Model file for the job. Use its own axes, mm. A direction names the side the tool comes from. Round coordinates to 2 decimals unless told otherwise and drop trailing zeros. Loops run counter-clockwise (first coordinate to the right, second up) from the corner with the lowest first, then second, coordinate; pieces in that order, holes last. Notation, with made-up numbers: (75.5, 27.5) - (119.5, 27.5) arc R17 ccw to (119.5, 39.5) - close; hole circle Ø9 at (81.25, -26). An arc over 180 degrees is marked (long way). Answer as a JSON object with one key per item and string values.
from build123d import *

# Parameters (mm, degrees)
SKETCH1_R           = 2.5
BOSS_EXTRUDE1_DEPTH = 10
SKETCH2_R           = 5
BOSS_EXTRUDE2_DEPTH = 5
FILLET1_R           = 5


with BuildPart() as part:
    # Sketch1 → Boss-Extrude1 (new body)
    with BuildSketch(Plane(origin=(0, 0, 0), x_dir=(1, 0, 0), z_dir=(0, 1, 0))):
        with Locations(Location((0, 0, 0), (0, 0, 270))):
            Circle(SKETCH1_R)
    extrude(amount=-BOSS_EXTRUDE1_DEPTH)

    # Sketch2 → Boss-Extrude2 (add)
    with BuildSketch(Plane(origin=(0, 0, 0), x_dir=(1, 0, 0), z_dir=(0, 1, 0))):
        with Locations(Location((0, 0, 0), (0, 0, 270))):
            Circle(SKETCH2_R)
    extrude(amount=BOSS_EXTRUDE2_DEPTH)

    # Fillet1
    fillet1_edges = [part.edges().sort_by_distance(p)[0] for p in [
        (0, 5, -5),
    ]]
    fillet(fillet1_edges, radius=FILLET1_R - 0.0001)  # a hair under: the kernel refuses the full size


solid = part.part
1) Probe probe 1 along Y at (x, z) = (-4.25, -1.25); probe 2 along Y at (x, z) = (-3, -2.25); probe 3 along Z at (x, y) = (0.5, -1.75). List the from-to ranges inside material, lowest first.
Values follow:
{"probe 1": "0 to 2.32", "probe 2": "0 to 3.31", "probe 3": "-2.45 to 2.45"}
2) Tool access for faces 1 (the cylindrical face through (-2.44, -4.93, -0.54)), 2 (the flat face through (0, -10, 0)): list every direction of +Z, -Z, +X, -X, +Y, -Y with a clear straight run to the whole face (end or side of a thin tool).
Values follow:
{"face 1": "-Y", "face 2": "+Z, -Z, +X, -X, -Y"}
3) Drop flat-ended pins along their axis: P1, Ø1, axis at x = -4, y = -1, coming from the +Z side; P2, Ø6, axis at x = -1.5, y = -8, coming from the -Z side; P3, Ø1.5, axis at x = 3, z = -4, coming from the -Y side. Give the stop position or say it passes through.
Values follow:
{"P1": "through", "P2": "z = -2.5", "P3": "y = 0"}
4) Slice it at A-A on y = -1.5. List the corners of the cut face in (x, z).
Values follow:
{"outline": "circle Ø5 at (0, 0)"}
